Model file for the job. Use its own axes, mm. Coordinates: 2 decimals unless noted, no trailing zeros. Order: outer loops, then holes, each group sorted by start corner. A loop starts at its lowest first (then second) coordinate and runs counter-clockwise, first axis right, second up.
from build123d import *

# Parameters (mm, degrees)
CROQUIS1_R              = 2
CROQUIS1_R_2            = 6.198274882
CROQUIS1_R_3            = 4.419717803
SALIENTE_EXTRUIR1_DEPTH = 2


with BuildPart() as part:
    # Croquis1 → Saliente-Extruir1 (new body)
    with BuildSketch(Plane.XY):
        with BuildLine():
            Line((2268.277850574, 1595.161717739), (2286.209587358, 1595.161717739))
            ThreePointArc((2286.209587358, 1595.161717739), (2286.758807426, 1595.131461929), (2287.301380655, 1595.041060665))
            ThreePointArc((2287.301380655, 1595.041060665), (2347.39348888, 1585.799291159), (2408.182765081, 1584.733611347))
            ThreePointArc((2408.182765081, 1584.733611347), (2416.444223404, 1577.280241595), (2408.198435589, 1569.809538977))
            ThreePointArc((2408.198435589, 1569.809538977), (2347.38385613, 1568.613783021), (2287.284769189, 1559.236008449))
            ThreePointArc((2287.284769189, 1559.236008449), (2286.73687453, 1559.143781296), (2286.18213001, 1559.112911855))
            Line((2286.18213001, 1559.112911855), (2268.277850574, 1559.112911855))
            ThreePointArc((2268.277850574, 1559.112911855), (2265.449423449, 1560.284484731), (2264.277850574, 1563.112911855))
            Line((2264.277850574, 1563.112911855), (2264.277850574, 1591.161717739))
            ThreePointArc((2264.277850574, 1591.161717739), (2265.449423449, 1593.990144863), (2268.277850574, 1595.161717739))
        make_face()
        with Locations((2272.325487006, 1587.265174947)):
            Circle(CROQUIS1_R, mode=Mode.SUBTRACT)
        with Locations((2408.944227539, 1577.272366482)):
            Circle(CROQUIS1_R, mode=Mode.SUBTRACT)
        with Locations((2272.360522717, 1567.00968004)):
            Circle(CROQUIS1_R, mode=Mode.SUBTRACT)
        with Locations((2285.218970732, 1577.142453031)):
            Circle(CROQUIS1_R_2, mode=Mode.SUBTRACT)
        with Locations((2300.394517149, 1577.158387592)):
            Circle(CROQUIS1_R_2, mode=Mode.SUBTRACT)
        with Locations((2315.570063567, 1577.174322153)):
            Circle(CROQUIS1_R_2, mode=Mode.SUBTRACT)
        with Locations((2330.745609984, 1577.190256713)):
            Circle(CROQUIS1_R_3, mode=Mode.SUBTRACT)
    extrude(amount=SALIENTE_EXTRUIR1_DEPTH)


solid = part.part
Q1. Cut at A-A, the plane z = 0.4. List the corners of the cut face in (x, y), plus the area to 3 significant figures.
Established:
outline: (2264.28, 1563.11) arc R4 ccw to (2268.28, 1559.11) - (2286.18, 1559.11) arc R5 ccw to (2287.28, 1559.24) arc R450.47 cw to (2408.2, 1569.81) arc R7.5 ccw (long way) to (2408.18, 1584.73) arc R450.47 cw to (2287.3, 1595.04) arc R5 ccw to (2286.21, 1595.16) - (2268.28, 1595.16) arc R4 ccw to (2264.28, 1591.16) - close; hole circle Ø4 at (2272.33, 1587.27); hole circle Ø4 at (2272.36, 1567.01); hole circle Ø12.4 at (2285.22, 1577.14); hole circle Ø12.4 at (2300.39, 1577.16); hole circle Ø12.4 at (2315.57, 1577.17); hole circle Ø8.84 at (2330.75, 1577.19); hole circle Ø4 at (2408.94, 1577.27)
area: 2,860 mm2
Q2. Probe line 1 (X direction, y = 1576, z = 1.6); line 2 (X direction, y = 1575, z = 1.55); line 3 (Y direction, x = 2409, z = 1.6). List the from-to ranges inside material, lowest first.
Established:
line 1: x = 2264.28 to 2279.13, 2291.31 to 2294.31, 2306.48 to 2309.48, 2321.66 to 2326.49, 2335 to 2407.4, 2410.49 to 2416.34
line 2: x = 2264.28 to 2279.4, 2291.04 to 2294.58, 2306.2 to 2309.77, 2321.37 to 2326.91, 2334.58 to 2416.09
line 3: y = 1569.77 to 1575.27, 1579.27 to 1584.77
Q3. Mould opens along Y. For faces 1 (the face through (2325, 1577, 0)), 2 (the face through (2334.83, 1575.5, 0.99)), 3 (the face through (2265.42, 1593.96, 0.99)) say: pulls with the +Y half, pulls with the -Y half, needs draft (parallel to the pull), parting line crosses it, or undercut.
Established:
face 1: needs draft
face 2: undercut
face 3: pulls with the +Y half
Q4. Cut at B-B, the plane x = 2388.5. List the corners of the cut face in (y, z).
Established:
outline: (1570.32, 0) - (1584.18, 0) - (1584.18, 2) - (1570.32, 2) - close
Q5. Drop flat-ended pins along their axis: P1, Ø1, axis at y = 1584.5, z = 0.5, coming from the +X side; P2, Ø1, axis at y = 1583, z = 1, coming from the +X side. Give the stop position or say it passes through.
Established:
P1: stops at x = 2412.26
P2: stops at x = 2414.32
